Autodesk Inventor part; units mm, degrees
ref_plane "YZ Plane" through (0, 0, 0) normal (1, 0, 0) x (0, 1, 0)
ref_plane "XZ Plane" through (0, 0, 0) normal (0, 1, 0) x (-1, 0, 0)
ref_plane "XY Plane" through (0, 0, 0) normal (0, 0, 1) x (1, 0, 0)
sketch "Эскиз1" plane through (0, 0, 0) normal (0, 0, 1) x (1, 0, 0)
  circle A0 centre (0, 0) radius 8.5
  circle A1 centre (0, 0) radius 3
  dimension "d0" = 6
  dimension "d1" = 17
extrude "Выдавливание1" add sketch "Эскиз1" along normal mid plane 6
chamfer "Фаска1" distance 0.5 angle 45 4 edges at (-8.5, 0, -3) (-8.5, 0, 3) (-3, 0, 3) (-3, 0, -3)
sketch "Эскиз2" plane through (0, 0, 3) normal (0, 0, 1) x (1, 0, 0)
  circle A0 centre (0, 0) radius 7.4
  circle A1 centre (0, 0) radius 4.4
  dimension "d7" = 8.8
  dimension "d8" = 14.8
extrude "Выдавливание2" cut sketch "Эскиз2" against normal blind 0.5
mirror "Зеркальное отражение1" about plane through (0, 0, 0) normal (0, 0, 1) of "Выдавливание2"
properties part number "Подшипник"
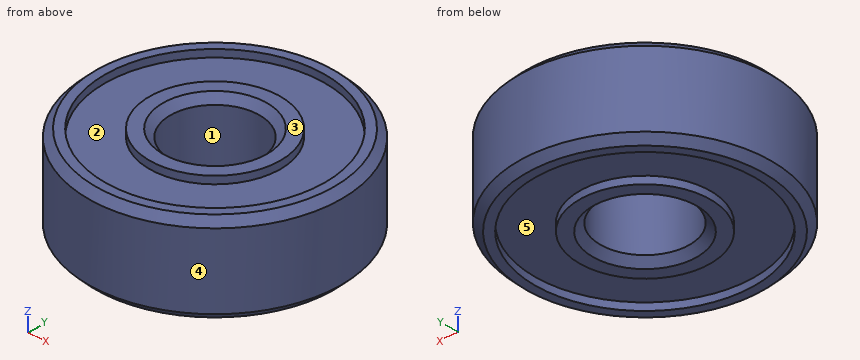
Geometry check sheet. Reference: the model listing, model coordinates, mm. Face numbers are marked on the shaded views. A direction names the side the tool comes from. Coordinates: 2 decimals unless noted, no trailing zeros. Order: outer loops, then holes, each group sorted by start corner. A loop starts at its lowest first (then second) coordinate and runs counter-clockwise, first axis right, second up. Notation, with made-up numbers: (81, -35) -> (125, -35) arc R23 ccw to (125, -13) -> close; hole circle Ø11 at (-3, 16). An arc over 180 degrees is marked (long way). Use a Markdown table: item, result. Add a question column.
1. Cross-section at C-C (z = 1.75). Enter the section's corners in (x, y), and give its area (3 significant figures).
2. Material ranges on L1, parallel to Y at x = 0, z = 0.55; L2, parallel to X at y = -3.25, z = -2.6; L3, parallel to Y at x = 0, z = -2.75, recorded low to high.
3. Go/stop test with flat-tipped pins: pin 1 Ø9.5 at (x, y) = (0, 0) entering from -Z; pin 2 Ø1 at (y, z) = (4.5, -1) entering from +X. Record where each tip stops, or that it passes through.
4. Set-up check for the marked faces 1 and 2: record each of +Z, -Z, +X, -X, +Y, -Y from which the full face is reachable in a straight line by a thin tool's end or side.
5. Mould release check, pull along X, two halves, no side actions. Record for the marked faces 3, 4 and 5: pulls with the +X half, pulls with the -X half, needs draft (parallel to the pull), parting line crosses it, or undercut.
Filled sheet:
| question | item | result |
|---|---|---|
| 1 | outline | circle Ø17 at (0, 0); hole circle Ø6 at (0, 0) |
| 1 | area | 199 mm2 |
| 2 | L1 | -8.5 to -3, 3 to 8.5 |
| 2 | L2 | -7.75 to -6.65, -2.97 to 2.97, 6.65 to 7.75 |
| 2 | L3 | -8.25 to -7.4, -4.4 to -3.25, 3.25 to 4.4, 7.4 to 8.25 |
| 3 | pin 1 | z = -3 |
| 3 | pin 2 | x = 7.5 |
| 4 | face 1 | +Z, -Z |
| 4 | face 2 | +Z |
| 5 | face 3 | needs draft |
| 5 | face 4 | parting line crosses it |
| 5 | face 5 | undercut |
